from build123d import *

# Parameters (mm, degrees)
BOSS_EXTRUDE1_DEPTH = 6
SKETCH1_3_R         = 1.5
SKETCH1_3_R_2       = 2.5
CUT_EXTRUDE1_DEPTH  = 6
SKETCH1_4_R         = 1.5
SKETCH1_4_R_2       = 2.5
CUT_EXTRUDE3_DEPTH  = 6


with BuildPart() as part:
    # Sketch1 → Boss-Extrude1 (new body)
    with BuildSketch(Plane(origin=(0, 0, 0), x_dir=(1, 0, 0), z_dir=(0, 1, 0))):
        Polygon((-125.323936458, 130.11669536), (-125.323936458, -44.88330464), (124.675630024, -44.88330464), (124.675630024, 44.651121259), (-45.323936458, 44.651121259), (-45.323936458, 130.11669536), align=None)
    extrude(amount=BOSS_EXTRUDE1_DEPTH)

    # Sketch1_3 → Cut-Extrude1 (cut)
    with BuildSketch(Plane(origin=(0, 0, 0), x_dir=(1, 0, 0), z_dir=(0, 1, 0))):
        with Locations((-100.323936458, 19)):
            Circle(SKETCH1_3_R)
        with Locations((-51.323936458, 19)):
            Circle(SKETCH1_3_R)
        with Locations((-51.323936458, -39)):
            Circle(SKETCH1_3_R)
        with Locations((-100.323936458, -39)):
            Circle(SKETCH1_3_R)
        with Locations((-115.323936458, 123.11669536)):
            Circle(SKETCH1_3_R_2)
    extrude(amount=CUT_EXTRUDE1_DEPTH, mode=Mode.SUBTRACT)

    # Sketch1_4 → Cut-Extrude3 (cut)
    with BuildSketch(Plane(origin=(0, 0, 0), x_dir=(1, 0, 0), z_dir=(0, 1, 0))):
        with Locations((4.675630024, 30.5)):
            Circle(SKETCH1_4_R)
        with Locations((99.675630024, 30.5)):
            Circle(SKETCH1_4_R)
        with Locations((99.675630024, -30.5)):
            Circle(SKETCH1_4_R)
        with Locations((4.675630024, -30.5)):
            Circle(SKETCH1_4_R)
        with Locations((-115.323936458, 38.11669536)):
            Circle(SKETCH1_4_R_2)
        with Locations((-115.323936458, -37.88330464)):
            Circle(SKETCH1_4_R_2)
        with Locations((114.675630024, -37.88330464)):
            Circle(SKETCH1_4_R_2)
        with Locations((114.675630024, 38.11669536)):
            Circle(SKETCH1_4_R_2)
    extrude(amount=CUT_EXTRUDE3_DEPTH, mode=Mode.SUBTRACT)


solid = part.part
For this review, take the finished solid that the model builds, in its own axes (mm). A direction names the side the tool comes from. Coordinates: 2 decimals unless noted, no trailing zeros. Order: outer loops, then holes, each group sorted by start corner. A loop starts at its lowest first (then second) coordinate and runs counter-clockwise, first axis right, second up. Notation, with made-up numbers: (66, 80.5) -> (95, 80.5) arc R22 ccw to (95, 92.5) -> close; hole circle Ø2 at (82.25, 69). An arc over 180 degrees is marked (long way). Return JSON: item names as keys, results as strings.
1. Machinability: for faces 1 (the flat face through (41, 3, -44.651)), 2 (the flat face through (-125.324, 3, -44)), which of the approach directions +Z, -Z, +X, -X, +Y, -Y give a long, thin tool a straight path to every point of the face, cutting with its end or side? Answer none if there is none.
Answer block:
{"face 1": "-Z, +X, +Y, -Y", "face 2": "+Z, -Z, -X, +Y, -Y"}
2. For line 1 (X direction, y = 4.35, z = -19); line 2 (X direction, y = 2.8, z = 30.5); line 3 (Z direction, x = 96, y = 4.9), list the stretches that pass through material, from the lowest coordinate up. Write a range as from..to.
Answer block:
{"line 1": "-125.32..-101.82, -98.82..-52.82, -49.82..124.68", "line 2": "-125.32..3.18, 6.18..98.18, 101.18..124.68", "line 3": "-44.65..44.88"}
3. We need section A-A on y = 3.35. State how many separate pieces and enclosed holes the cut face has, and give its area (3 significant figures).
Answer block:
{"separate pieces": "1", "enclosed holes": "13", "area": "29,100 mm²"}
4. The part is to be moulded in two halves that separate along Z. For faces 3 (the cylindrical face through (-114.17, 2.96, 40.1)), 4 (the flat face through (-85, 3, -130.117)), 5 (the flat face through (-30, 6, -24)), 6 (the cylindrical face through (115.83, 2.96, 40.1)), say which applies: +Z half, -Z half, draft (parallel to the pull), parting line (faces both ways), or undercut.
Answer block:
{"face 3": "undercut", "face 4": "-Z half", "face 5": "draft", "face 6": "undercut"}
5. For pin 1 Ø5 at (x, z) = (4.68, -30.5) entering from -Y; pin 2 Ø1.8 at (y, z) = (3.5, -93) entering from +X; pin 3 Ø3 at (x, y) = (13.5, 3) entering from -Z, all flat-tipped, find the tip position at first contact; note any pin that passes through.
Answer block:
{"pin 1": "y = 0", "pin 2": "x = -45.32", "pin 3": "z = -44.65"}
6. We need section B-B on x = 36. Write out the cut boundary in (y, z).
Answer block:
{"outline": "(0, -44.65) -> (6, -44.65) -> (6, 44.88) -> (0, 44.88) -> close"}
7. We need section C-C on z = -61.5. Write out the cut boundary in (x, y), and give its area (3 significant figures).
Answer block:
{"outline": "(-125.32, 0) -> (-45.32, 0) -> (-45.32, 6) -> (-125.32, 6) -> close", "area": "480 mm²"}
